```python
from build123d import *

# Parameters (mm, degrees)
SKETCH1_R           = 21.5
BOSS_EXTRUDE1_DEPTH = 160
CUT_EXTRUDE1_START  = -20
CUT_EXTRUDE1_DEPTH  = 20
SKETCH4_R           = 15
BOSS_EXTRUDE2_DEPTH = 26
CHAMFER1_SIZE       = 2


with BuildPart() as part:
    # Sketch1 → Boss-Extrude1 (new body)
    with BuildSketch(Plane(origin=(0, 0, 0), x_dir=(1, 0, 0), z_dir=(0, 1, 0))):
        with Locations(Location((0, 0, 0), (0, 0, 270))):
            Circle(SKETCH1_R)
    extrude(amount=-BOSS_EXTRUDE1_DEPTH)

    # Sketch3 → Cut-Extrude1 (cut)
    with BuildSketch(Plane.XZ.offset(160).offset(CUT_EXTRUDE1_START)):
        with BuildLine():
            Line((-4, 17.036725037), (-4, 21.124630174))
            ThreePointArc((-4, 21.124630174), (-10.75, 18.619546181), (-16.294466376, 14.026416702))
            Line((-16.294466376, 14.026416702), (-12.75423668, 11.982464134))
            ThreePointArc((-12.75423668, 11.982464134), (-8.75, 15.155444566), (-4, 17.036725037))
        make_face()
        with BuildLine():
            ThreePointArc((16.294466376, 14.026416702), (10.75, 18.619546181), (4, 21.124630174))
            Line((4, 21.124630174), (4, 17.036725037))
            ThreePointArc((4, 17.036725037), (8.75, 15.155444566), (12.75423668, 11.982464134))
            Line((12.75423668, 11.982464134), (16.294466376, 14.026416702))
        make_face()
        with BuildLine():
            ThreePointArc((21.5, 0), (21.196474083, 3.599928673), (20.294466376, 7.098213472))
            Line((20.294466376, 7.098213472), (16.75423668, 5.054260904))
            ThreePointArc((16.75423668, 5.054260904), (17.5, 0), (16.75423668, -5.054260904))
            Line((16.75423668, -5.054260904), (20.294466376, -7.098213472))
            ThreePointArc((20.294466376, -7.098213472), (21.196474083, -3.599928673), (21.5, 0))
        make_face()
        with BuildLine():
            Line((-16.75423668, 5.054260904), (-20.294466376, 7.098213472))
            ThreePointArc((-20.294466376, 7.098213472), (-21.5, 0), (-20.294466376, -7.098213472))
            Line((-20.294466376, -7.098213472), (-16.75423668, -5.054260904))
            ThreePointArc((-16.75423668, -5.054260904), (-17.5, 0), (-16.75423668, 5.054260904))
        make_face()
        with BuildLine():
            Line((-12.75423668, -11.982464134), (-16.294466376, -14.026416702))
            ThreePointArc((-16.294466376, -14.026416702), (-10.75, -18.619546181), (-4, -21.124630174))
            Line((-4, -21.124630174), (-4, -17.036725037))
            ThreePointArc((-4, -17.036725037), (-8.75, -15.155444566), (-12.75423668, -11.982464134))
        make_face()
        with BuildLine():
            Line((4, -17.036725037), (4, -21.124630174))
            ThreePointArc((4, -21.124630174), (10.75, -18.619546181), (16.294466376, -14.026416702))
            Line((16.294466376, -14.026416702), (12.75423668, -11.982464134))
            ThreePointArc((12.75423668, -11.982464134), (8.75, -15.155444566), (4, -17.036725037))
        make_face()
    extrude(amount=CUT_EXTRUDE1_DEPTH, mode=Mode.SUBTRACT)

    # Sketch4 → Boss-Extrude2 (add)
    with BuildSketch(Plane.XZ.offset(160)):
        with Locations(Location((0, 0, 0), (0, 0, 90))):
            Circle(SKETCH4_R)
    extrude(amount=BOSS_EXTRUDE2_DEPTH)

    # Chamfer1
    chamfer1_edges = [part.edges().sort_by_distance(p)[0] for p in [
        (0, -186, -15),
    ]]
    chamfer(chamfer1_edges, length=CHAMFER1_SIZE)


solid = part.part
```
Here's how the part is built. I have some questions about the finished solid (model axes, mm). A direction names the side the tool comes from. Round coordinates to 2 decimals unless told otherwise and drop trailing zeros. Order: outer loops, then holes, each group sorted by start corner. A loop starts at its lowest first (then second) coordinate and runs counter-clockwise, first axis right, second up. Notation, with made-up numbers: M 7,41 L 35,41 A16 ccw 35,61 Z; hole C -23,-29.5 d2. An arc over 180 degrees is marked long. One line per question, with ' | ' between items.
1) I want a section at B-B, the plane x = 0. Write out the boundary of the cut face in (y, z).
Working result:
outline: M -186,-13 L -184,-15 L -160,-15 L -160,-21.5 L 0,-21.5 L 0,21.5 L -160,21.5 L -160,15 L -184,15 L -186,13 Z
2) I want a section at A-A, the plane z = 0. Write out the boundary of the cut face in (x, y), then the cut area to 3 significant figures.
Working result:
outline: M -21.5,-140 L -17.5,-140 L -17.5,-160 L -15,-160 L -15,-184 L -13,-186 L 13,-186 L 15,-184 L 15,-160 L 17.5,-160 L 17.5,-140 L 21.5,-140 L 21.5,0 L -21.5,0 Z | area: 7,500 mm²
3) I want a section at C-C, the plane y = -167. Write out the boundary of the cut face in (x, z), then the cut area to 3 significant figures.
Working result:
outline: C 0,0 d30 | area: 707 mm²
4) For pin 1 Ø2 at (y, z) = (-150.5, 20) entering from -X; pin 2 Ø7.5 at (x, z) = (-13, 14.5) entering from -Y; pin 3 Ø2 at (x, y) = (-14, -165.5) entering from -Z, each with a flat end and sliding along its axis, tell me the tip position at first contact or that it passes through.
Working result:
pin 1: x = -4 | pin 2: y = -160 | pin 3: z = -7.48
5) I want a section at D-D, the plane y = -94. Write out the boundary of the cut face in (x, z), then the cut area to 3 significant figures.
Working result:
outline: C 0,0 d43 | area: 1,450 mm²
6) I need wall thicknesses on line 1 along Y through (x, z) = (1, 15); line 2 along Y through (x, z) = (-13, -17); line 3 along X through (y, z) = (-133.5, 0). Which ranges of each line are inside material? Lowest first, please.
Working result:
line 1: -160 to 0 | line 2: -140 to 0 | line 3: -21.5 to 21.5
7) If we mould it in two halves opening along Z, with no side actions, what happens to faces 1 (the face through (-18.55, -149.86, -6.09)), 2 (the face through (-0.66, -171.832, -14.985)), 3 (the face through (15.1, -160, 1.5))? For each: +Z half, -Z half, draft (parallel to the pull), parting line (faces both ways), or undercut.
Working result:
face 1: undercut | face 2: parting line | face 3: draft
8) For faces 4 (the face through (-18.5, -149.86, 6.06)), 5 (the face through (-4, -150, -19)), 6 (the face through (-8.81, -149.86, 15.12)), 7 (the face through (-14.5, -149.86, -12.99)), which set-ups out of +Z, -Z, +X, -X, +Y, -Y let a thin tool reach every point of the face, with its end or its side?
Working result:
face 4: -X, -Y | face 5: -Z, -X, -Y | face 6: +Z, -Y | face 7: -Z, -Y
